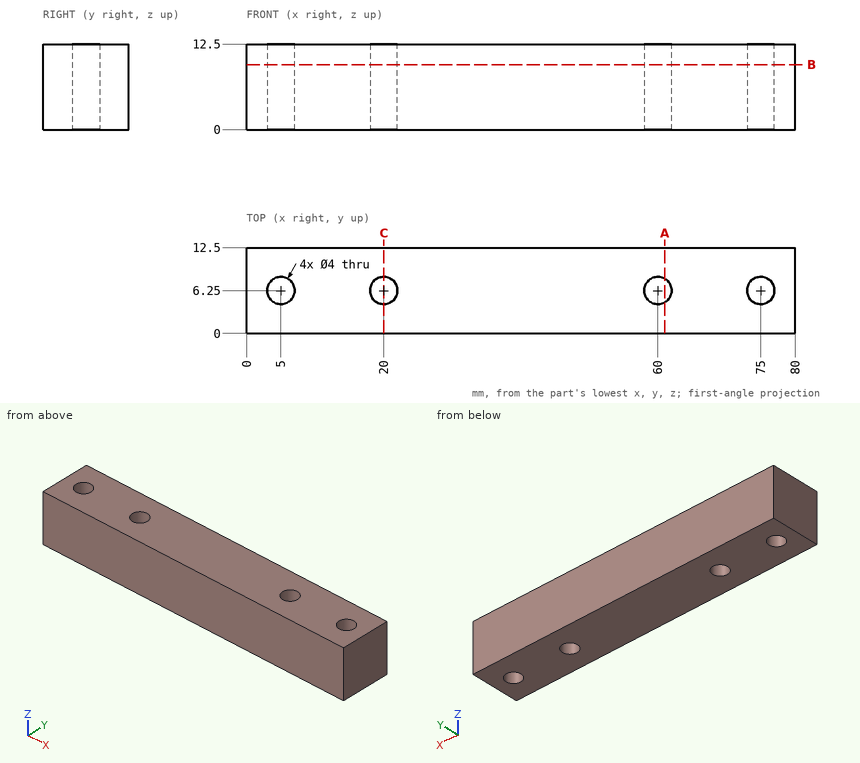
The figure shows three views and two pictorial views of one solid part (mm, origin at its lowest corner). Answer the questions. Give positions to 0.01 mm unless a question says otherwise; leave off trailing zeros. Order: outer loops, then holes, each group sorted by start corner. A loop starts at its lowest first (then second) coordinate and runs counter-clockwise, first axis right, second up. Notation, with made-up numbers: M 84,-2.5 L 105,-2.5 A7 ccw 105,3.5 Z; hole C 4.25,61.5 d1. An arc over 180 degrees is marked long. Return JSON: item names as keys, results as strings.
Q1. Find the intervals of material crossed by line 1 along X through (y, z) = (6.25, 7.25); line 2 along Y through (x, z) = (20, 7.5); line 3 along X through (y, z) = (7.25, 3.25), in increasing order. Write a range as [from, to].
Answer below:
{"line 1": "x = [0, 3], [7, 18], [22, 58], [62, 73], [77, 80]", "line 2": "y = [0, 4.25], [8.25, 12.5]", "line 3": "x = [0, 3.27], [6.73, 18.27], [21.73, 58.27], [61.73, 73.27], [76.73, 80]"}
Q2. Find section C-C, the plane x = 20. Write down the section's boundary in (y, z), and give its area (3 significant figures).
Answer below:
{"outline": "M 0,0 L 4.25,0 L 4.25,12.5 L 0,12.5 Z; M 8.25,0 L 12.5,0 L 12.5,12.5 L 8.25,12.5 Z", "area": "106 mm^2"}
Q3. Find section B-B, the plane z = 9.5. Write down the section's boundary in (x, y).
Answer below:
{"outline": "M 0,0 L 80,0 L 80,12.5 L 0,12.5 Z; hole C 5,6.25 d4; hole C 20,6.25 d4; hole C 60,6.25 d4; hole C 75,6.25 d4"}
Q4. This flat-tipped pin is pushed along its axis until it touches: pin 1 (2.5 mm diameter, centred on x = 20, y = 6.25, fed in from +Z). Where does it stop, or does it pass through?
Answer below:
{"pin 1": "passes through"}
Q5. Find section A-A, the plane x = 61. Write down the section's boundary in (y, z).
Answer below:
{"outline": "M 0,0 L 4.52,0 L 4.52,12.5 L 0,12.5 Z; M 7.98,0 L 12.5,0 L 12.5,12.5 L 7.98,12.5 Z"}
